Could you check a few things on this drawing? It's one solid part, dimensions in mm from its lowest x, y, z. A direction names the side the tool comes from. Coordinates: 2 decimals unless noted, no trailing zeros. Write each loop counter-clockwise with the first axis right and the second up, starting at its lowest first coordinate (ties: lowest second). Pieces come first, ordered by that corner, then holes. Notation, with made-up numbers: (63.5, 43.5) - (112.5, 43.5) arc R17 ccw to (112.5, 66.5) - close; hole circle Ø1 at (-26.75, -32.75). An arc over 180 degrees is marked (long way). Answer as a JSON object with one key per item and string values. Group by question number.
1) We'd pull the mould along X, two halves only. Please class the marked faces 1, 2, 3 and 4: released by +X, released by -X, zero draft, split by the parting line, or undercut.
2) If we section it at A-A (z = 10): Write out the boundary of the cut face in (x, y).
3) Please list where these lines run through material, in increasing order: line 1 along Z through (x, y) = (40, 88.65); line 2 along Y through (x, z) = (24.5, 18); line 3 along X through (y, z) = (62, 29.5).
4) If we section it at B-B (y = 41.5): Write out the boundary of the cut face in (x, z).
5) If we section it at D-D (y = 32.3): Write out the boundary of the cut face in (x, z).
6) On a 3-axis mill with a long thin cutter (end or side, diameter ignored), from which of +Z, -Z, +X, -X, +Y, -Y can I reach the whole of each face in a straight line? I mean the marked faces 5 and 6. Say none if no direction works.
7) Will this pin go through, and if not, where does the flat tip stop? pin 1 Ø14.5 at (x, z) = (28, 36) entering from -Y.
8) If we section it at C-C (x = 40): Write out the boundary of the cut face in (y, z), plus the area to 3 significant figures.
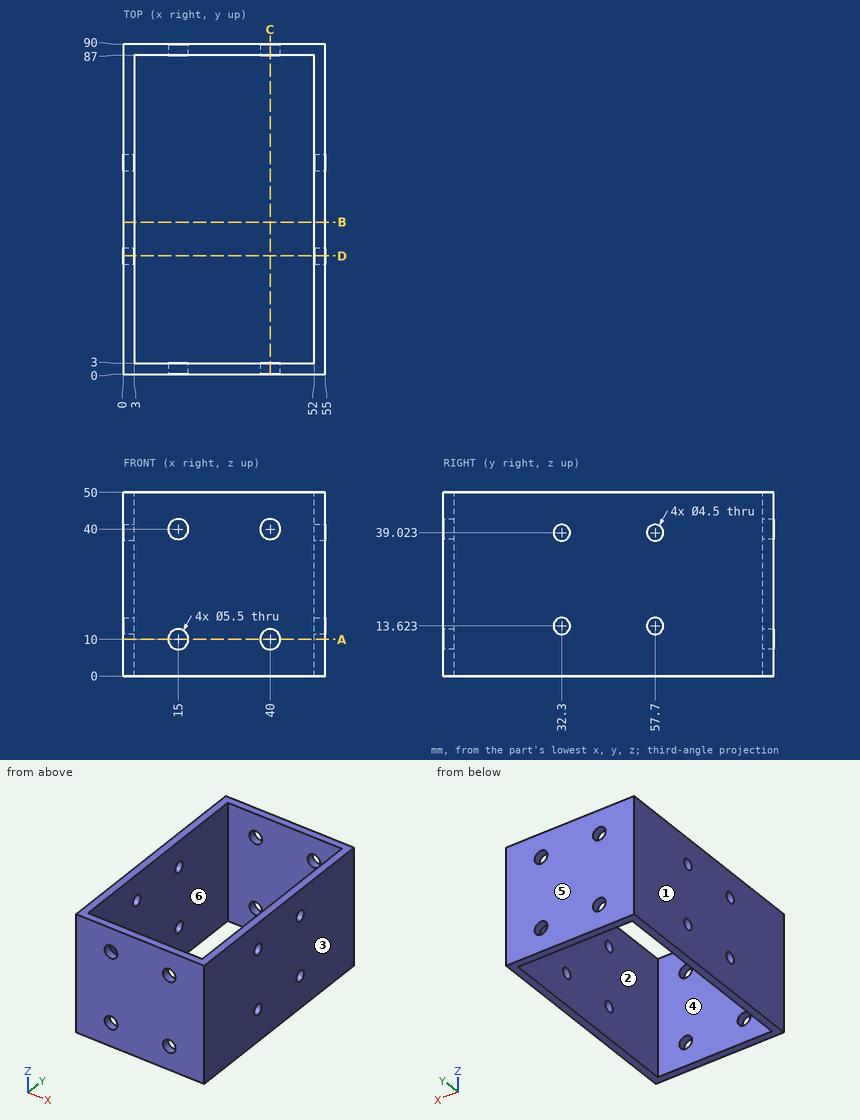
Here are the results:
{
 "1": {"face 1": "released by -X", "face 2": "undercut", "face 3": "released by +X", "face 4": "undercut"},
 "2": {"outline": "(0, 0) - (12.25, 0) - (12.25, 3) - (3, 3) - (3, 87) - (12.25, 87) - (12.25, 90) - (0, 90) - close; (17.75, 0) - (37.25, 0) - (37.25, 3) - (17.75, 3) - close; (17.75, 87) - (37.25, 87) - (37.25, 90) - (17.75, 90) - close; (42.75, 0) - (55, 0) - (55, 90) - (42.75, 90) - (42.75, 87) - (52, 87) - (52, 3) - (42.75, 3) - close"},
 "3": {"line 1": "z = 0 to 7.25, 12.75 to 37.25, 42.75 to 50", "line 2": "y = 0 to 3, 87 to 90", "line 3": "x = 0 to 3, 52 to 55"},
 "4": {"outline": "(0, 0) - (3, 0) - (3, 50) - (0, 50) - close; (52, 0) - (55, 0) - (55, 50) - (52, 50) - close"},
 "5": {"outline": "(0, 0) - (3, 0) - (3, 11.37) - (0, 11.37) - close; (0, 15.87) - (3, 15.87) - (3, 36.77) - (0, 36.77) - close; (0, 41.27) - (3, 41.27) - (3, 50) - (0, 50) - close; (52, 0) - (55, 0) - (55, 11.37) - (52, 11.37) - close; (52, 15.87) - (55, 15.87) - (55, 36.77) - (52, 36.77) - close; (52, 41.27) - (55, 41.27) - (55, 50) - (52, 50) - close"},
 "6": {"face 5": "+Z, -Z, +X, -X, +Y", "face 6": "+Z, -Z"},
 "7": {"pin 1": "stops at y = 0"},
 "8": {"outline": "(0, 0) - (3, 0) - (3, 7.25) - (0, 7.25) - close; (0, 12.75) - (3, 12.75) - (3, 37.25) - (0, 37.25) - close; (0, 42.75) - (3, 42.75) - (3, 50) - (0, 50) - close; (87, 0) - (90, 0) - (90, 7.25) - (87, 7.25) - close; (87, 12.75) - (90, 12.75) - (90, 37.25) - (87, 37.25) - close; (87, 42.75) - (90, 42.75) - (90, 50) - (87, 50) - close", "area": "234 mm²"}
}
